from build123d import *

# Parameters (mm, degrees)
SKETCH1_W           = 115
SKETCH1_H           = 75
SKETCH1_R           = 6
BOSS_EXTRUDE1_DEPTH = 5
CUT_EXTRUDE1_DEPTH  = 5
FILLET1_R           = 20
SKETCH5_R           = 7.5
CUT_EXTRUDE4_DEPTH  = 10
SKETCH9_W           = 57.70776026
SKETCH9_H           = 31
CUT_EXTRUDE5_DEPTH  = 10
FILLET2_R           = 10
CUT_EXTRUDE7_DEPTH  = 16
FILLET3_R           = 1


with BuildPart() as part:
    # Sketch1 → Boss-Extrude1 (new body)
    with BuildSketch(Plane(origin=(0, 0, 0), x_dir=(1, 0, 0), z_dir=(0, 1, 0))):
        Rectangle(SKETCH1_W, SKETCH1_H)
        with Locations(Location((-44.48, 24.48, 0), (0, 0, 270))):
            Circle(SKETCH1_R, mode=Mode.SUBTRACT)
        with Locations(Location((44.48, -24.48, 0), (0, 0, 270))):
            Circle(SKETCH1_R, mode=Mode.SUBTRACT)
    extrude(amount=BOSS_EXTRUDE1_DEPTH)

    # Sketch2 → Cut-Extrude1 (cut)
    with BuildSketch(Plane(origin=(0, 5, 0), x_dir=(1, 0, 0), z_dir=(0, 1, 0))):
        with BuildLine():
            Line((-41.5, 15.5), (41.5, 15.5))
            ThreePointArc((41.5, 15.5), (48.571067812, 12.571067812), (51.5, 5.5))
            Line((51.5, 5.5), (51.5, -5.5))
            ThreePointArc((51.5, -5.5), (48.571067812, -12.571067812), (41.5, -15.5))
            Line((41.5, -15.5), (-41.5, -15.5))
            ThreePointArc((-41.5, -15.5), (-48.571067812, -12.571067812), (-51.5, -5.5))
            Line((-51.5, -5.5), (-51.5, 5.5))
            ThreePointArc((-51.5, 5.5), (-48.571067812, 12.571067812), (-41.5, 15.5))
        make_face()
    extrude(amount=-CUT_EXTRUDE1_DEPTH, mode=Mode.SUBTRACT)

    # Fillet1
    fillet1_edges = [part.edges().sort_by_distance(p)[0] for p in [
        (57.5, 2.5, 37.5),
        (-57.5, 2.5, 37.5),
        (-57.5, 2.5, -37.5),
        (57.5, 2.5, -37.5),
    ]]
    fillet(fillet1_edges, radius=FILLET1_R)

    # Sketch5 → Cut-Extrude4 (cut)
    with BuildSketch(Plane.XZ):
        with Locations(Location((-39.5, 25.5, 0), (0, 0, 270))):
            Circle(SKETCH5_R)
        with Locations(Location((39.5, -25.5, 0), (0, 0, 270))):
            Circle(SKETCH5_R)
    extrude(amount=-CUT_EXTRUDE4_DEPTH, mode=Mode.SUBTRACT)

    # Sketch9 → Cut-Extrude5 (cut)
    with BuildSketch(Plane(origin=(0, 5, 0), x_dir=(1, 0, 0), z_dir=(0, 1, 0))):
        Polygon((-35.360842569, 29.5), (-35.360842569, 15.5), (-28.606695745, 15.5), (29.101064515, 15.5), (29.101064515, 29.5), align=None)
        Polygon((-28.606695745, 15.5), (-35.360842569, 15.5), (-52.5, 15.5), (-52.5, -15.5), (-28.606695745, -15.5), align=None)
        with Locations((0.247184385, 0)):
            Rectangle(SKETCH9_W, SKETCH9_H)
        Polygon((52.5, 15.5), (29.101064515, 15.5), (29.101064515, -15.5), (36.173307785, -15.5), (52.5, -15.5), align=None)
        Polygon((29.101064515, -15.5), (-28.606695745, -15.5), (-28.606695745, -29.5), (36.173307785, -29.5), (36.173307785, -15.5), align=None)
    extrude(amount=-CUT_EXTRUDE5_DEPTH, mode=Mode.SUBTRACT)

    # Fillet2
    fillet2_edges = [part.edges().sort_by_distance(p)[0] for p in [
        (-35.360842569, 2.5, -15.5),
        (29.101064515, 2.5, -15.5),
        (36.173307785, 2.5, 15.5),
        (-28.606695745, 2.5, 15.5),
    ]]
    fillet(fillet2_edges, radius=FILLET2_R)

    # Sketch11 → Cut-Extrude7 (cut)
    with BuildSketch(Plane(origin=(0, 5, 0), x_dir=(1, 0, 0), z_dir=(0, 1, 0))):
        with BuildLine():
            Line((57.5, -17.5), (57.5, 17.5))
            ThreePointArc((57.5, 17.5), (51.642135624, 31.642135624), (37.5, 37.5))
            Line((37.5, 37.5), (-37.5, 37.5))
            ThreePointArc((-37.5, 37.5), (-51.642135624, 31.642135624), (-57.5, 17.5))
            Line((-57.5, 17.5), (-57.5, -17.5))
            ThreePointArc((-57.5, -17.5), (-51.642135624, -31.642135624), (-37.5, -37.5))
            Line((-37.5, -37.5), (37.5, -37.5))
            ThreePointArc((37.5, -37.5), (51.642135624, -31.642135624), (57.5, -17.5))
        make_face()
        with BuildLine():
            Line((37.5, 36.5), (-37.5, 36.5))
            ThreePointArc((-37.5, 36.5), (-50.935028843, 30.935028843), (-56.5, 17.5))
            Line((-56.5, 17.5), (-56.5, -17.5))
            ThreePointArc((-56.5, -17.5), (-50.935028843, -30.935028843), (-37.5, -36.5))
            Line((-37.5, -36.5), (37.5, -36.5))
            ThreePointArc((37.5, -36.5), (50.935028843, -30.935028843), (56.5, -17.5))
            Line((56.5, -17.5), (56.5, 17.5))
            ThreePointArc((56.5, 17.5), (50.935028843, 30.935028843), (37.5, 36.5))
        make_face(mode=Mode.SUBTRACT)
    extrude(amount=-CUT_EXTRUDE7_DEPTH, mode=Mode.SUBTRACT)

    # Fillet3
    fillet3_edges = [part.edges().sort_by_distance(p)[0] for p in [
        (52.5, 5, 0),
        (3.78330602, 5, 29.5),
        (-52.5, 0, 0),
        (-3.129889027, 0, -29.5),
        (-3.129889027, 5, -29.5),
        (-52.5, 5, 0),
        (36.173307785, 0, 27.5),
        (36.173307785, 5, 27.5),
        (29.101064515, 0, -27.5),
        (-35.360842569, 0, -27.5),
        (-48.930421284, 0, -15.5),
        (-28.606695745, 0, 27.5),
        (49.336653893, 0, 15.5),
        (32.029996703, 0, -18.428932188),
        (-38.289774757, 0, -18.428932188),
        (-31.535627933, 0, 18.428932188),
        (39.102239973, 0, 18.428932188),
        (49.336653893, 5, 15.5),
        (29.101064515, 5, -27.5),
        (-28.606695745, 5, 27.5),
        (-48.930421284, 5, -15.5),
        (-35.360842569, 5, -27.5),
        (32.029996703, 5, -18.428932188),
        (-38.289774757, 5, -18.428932188),
        (-31.535627933, 5, 18.428932188),
        (39.102239973, 5, 18.428932188),
        (0, 0, -36.5),
        (-50.935028843, 0, -30.935028843),
        (-56.5, 0, 0),
        (-50.935028843, 0, 30.935028843),
        (0, 0, 36.5),
        (50.935028843, 0, 30.935028843),
        (56.5, 0, 0),
        (50.935028843, 0, -30.935028843),
        (50.935028843, 5, -30.935028843),
        (56.5, 5, 0),
        (50.935028843, 5, 30.935028843),
        (0, 5, 36.5),
        (-50.935028843, 5, 30.935028843),
        (-56.5, 5, 0),
        (-50.935028843, 5, -30.935028843),
        (0, 5, -36.5),
        (-45.553347872, 0, 15.5),
        (45.800532257, 0, -15.5),
        (45.800532257, 5, -15.5),
        (-45.553347872, 5, 15.5),
        (52.5, 0, 0),
        (3.78330602, 0, 29.5),
    ]]
    fillet(fillet3_edges, radius=FILLET3_R)


solid = part.part
Build history of the part. All positions in model axes, mm. A direction names the side the tool comes from. Give positions to 0.01 mm unless a question says otherwise; leave off trailing zeros. Order: outer loops, then holes, each group sorted by start corner. A loop starts at its lowest first (then second) coordinate and runs counter-clockwise, first axis right, second up. Notation, with made-up numbers: M 65.25,14 L 88.25,14 A30 ccw 88.25,40 Z; hole C 50,78.5 d3. An arc over 180 degrees is marked long. Use one line per item in the form item = value.
1) Probe probe 1 along Z at (x, y) = (-1, 1.6); probe 2 along X at (y, z) = (1.5, 2.5); probe 3 along X at (y, z) = (3.65, -24.48). List the from-to ranges inside material, lowest first.
Calculated:
probe_1 = -36.5 to -29.5, 29.5 to 36.5
probe_2 = -56.5 to -52.5, 52.5 to 56.5
probe_3 = -55.17 to -50.48, -38.48 to -35.41, 29.15 to 32.07, 46.93 to 55.17
2) Drop flat-ended pins along their axis: pin 1 (2.5 mm diameter, centred on x = 43.5, y = 2, fed in from +Z); pin 2 (2.5 mm diameter, centred on y = 3, z = -28.5, fed in from -X); pin 3 (0.9 mm diameter, centred on y = 2.5, z = 27.5, fed in from +X). Give the stop position or say it passes through.
Calculated:
pin_1 = 35.9
pin_2 = -53.81
pin_3 = 53.93
3) Saw through at D-D (z = 21.5). State how many separate pieces and enclosed holes the cut face has, plus the area to 3 significant figures.
Calculated:
separate_pieces = 4
enclosed_holes = 0
area = 111 mm2
4) Saw through at B-B (z = 12.5). Give the cut face in (x, y).
Calculated:
outline = M -56.5,1 A1 ccw -55.5,0 L -53.5,0 A1 ccw -52.5,1 L -52.5,4 A1 ccw -53.5,5 L -55.5,5 A1 ccw -56.5,4 Z; M 52.5,1 A1 ccw 53.5,0 L 55.5,0 A1 ccw 56.5,1 L 56.5,4 A1 ccw 55.5,5 L 53.5,5 A1 ccw 52.5,4 Z
5) Saw through at A-A (x = -9.5). Give the cut face in (y, z), plus the area to 3 significant figures.
Calculated:
outline = M 0,-35.5 A1 ccw 1,-36.5 L 4,-36.5 A1 ccw 5,-35.5 L 5,-30.5 A1 ccw 4,-29.5 L 1,-29.5 A1 ccw 0,-30.5 Z; M 0,30.5 A1 ccw 1,29.5 L 4,29.5 A1 ccw 5,30.5 L 5,35.5 A1 ccw 4,36.5 L 1,36.5 A1 ccw 0,35.5 Z
area = 68.3 mm2
6) Saw through at C-C (y = 2.1). Give the cut face in (x, z).
Calculated:
outline = M -56.5,-17.5 A19 ccw -37.5,-36.5 L 37.5,-36.5 A19 ccw 56.5,-17.5 L 56.5,17.5 A19 ccw 37.5,36.5 L -37.5,36.5 A19 ccw -56.5,17.5 Z; hole M -52.5,-15.5 L -45.36,-15.5 A10 cw -35.36,-25.5 L -35.36,-29.5 L 29.1,-29.5 L 29.1,-25.5 A10 cw 39.1,-15.5 L 52.5,-15.5 L 52.5,15.5 L 46.17,15.5 A10 cw 36.17,25.5 L 36.17,29.5 L -28.61,29.5 L -28.61,25.5 A10 cw -38.61,15.5 L -52.5,15.5 Z; hole C -44.48,-24.48 d12; hole C -39.5,25.5 d15; hole C 39.5,-25.5 d15; hole C 44.48,24.48 d12
7) Two-plate mould, pull along X, no slides. Class faces 3 (the face through (-46, 3, 15.5)), 4 (the face through (1, 3, -36.5)), 5 (the face through (-56.5, 3, 0)), 6 (the face through (-31.614, 2.479, 18.352)): released by +X, released by -X, zero draft, split by the parting line, or undercut.
Calculated:
face_3 = undercut
face_4 = zero draft
face_5 = released by -X
face_6 = undercut
8) Tool access for faces 1 (the face through (-4, 5, 31)), 2 (the face through (52.5, 3, 0)): list every direction of +Z, -Z, +X, -X, +Y, -Y with a clear straight run to the whole face (end or side of a thin tool).
Calculated:
face_1 = +Z, -Z, +X, -X, +Y
face_2 = +Y, -Y
